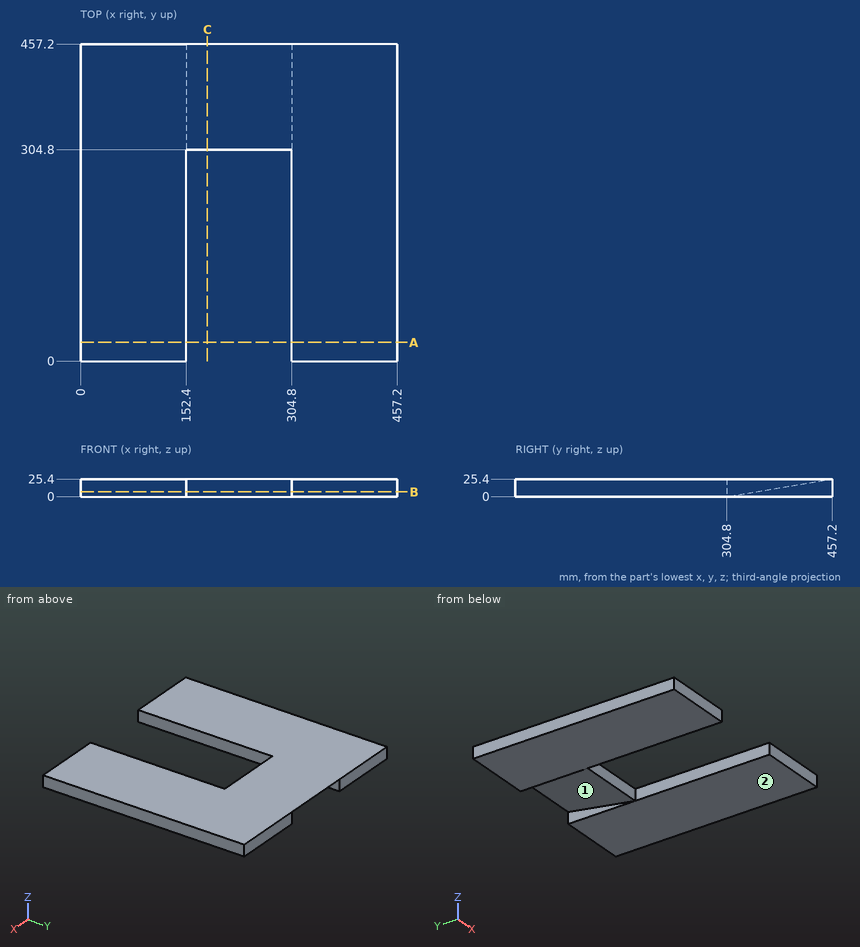
Input: dimensioned drawing with shaded views. Units: mm. Origin: part minimum x, y, z. Give positions to 0.01 mm unless a question says otherwise; leave off trailing zeros. Write each loop counter-clockwise with the first axis right and the second up, starting at its lowest first coordinate (ties: lowest second). Pieces come first, ordered by that corner, then holes. Notation, with made-up numbers: M -17,-21 L 32,-21 A17 ccw 32,8 Z; hole C -30.5,-29 d10. An arc over 180 degrees is marked long. Return JSON: item names as keys, results as strings. Group by question number.
1) Cut plane C-C, the plane x = 183. Output: boundary loops of the cut face in (y, z).
2) Material intervals for line 1 along X through (y, z) = (203, 5); line 2 along Z through (x, y) = (290, 369); line 3 along Z through (x, y) = (254.5, 415.5), sorted ascending. Write a range as [from, to].
3) Cut plane B-B, the plane z = 7. Output: boundary loops of the cut face in (x, y).
4) Pull-direction query (X, two-part tool) for the marked faces 1 and 2; classes: pulls with the +X half, pulls with the -X half, needs draft (parallel to the pull), parting line crosses it, or undercut.
5) Cut plane A-A, the plane y = 27. Output: boundary loops of the cut face in (x, z), plus the area to 3 significant figures.
Recorded:
{
 "1": {"outline": "M 304.8,0 L 457.2,25.4 L 304.8,25.4 Z"},
 "2": {"line 1": "x = [0, 152.4], [304.8, 457.2]", "line 2": "z = [10.7, 25.4]", "line 3": "z = [18.45, 25.4]"},
 "3": {"outline": "M 0,0 L 152.4,0 L 152.4,304.8 L 304.8,304.8 L 304.8,0 L 457.2,0 L 457.2,457.2 L 304.8,457.2 L 304.8,346.8 L 152.4,346.8 L 152.4,457.2 L 0,457.2 Z"},
 "4": {"face 1": "undercut", "face 2": "needs draft"},
 "5": {"outline": "M 0,0 L 152.4,0 L 152.4,25.4 L 0,25.4 Z; M 304.8,0 L 457.2,0 L 457.2,25.4 L 304.8,25.4 Z", "area": "7,740 mm²"}
}
